```python
from build123d import *

# Parameters (mm, degrees)
F0_R     = 17.018
F0_R_2   = 18.846805
F1_DEPTH = 2
F2_DEPTH = 25
F3_SIZE  = 0.5


with BuildPart() as f1:
    # F0 (on Front) → F1 (new body)
    with BuildSketch(Plane.XZ):
        Circle(F0_R)
        Circle(F0_R_2)
        Circle(F0_R, mode=Mode.SUBTRACT)
    extrude(amount=F1_DEPTH)

    # F0 (on Front) → F2 (cut)
    with BuildSketch(Plane.XZ):
        Circle(F0_R)
    extrude(amount=F2_DEPTH, mode=Mode.SUBTRACT)

    # F3
    f3_edges = [f1.edges().sort_by_distance(p)[0] for p in [
        (-18.846805, 0, 0),
    ]]
    chamfer(f3_edges, length=F3_SIZE)


solid = f1.part
```
Part model, mm, in its own coordinate system. Round coordinates to 2 decimals unless told otherwise and drop trailing zeros. Write each loop counter-clockwise with the first axis right and the second up, starting at its lowest first coordinate (ties: lowest second). Pieces come first, ordered by that corner, then holes. Notation, with made-up numbers: M -12,61 L -7,61 A10 cw -7,79 Z; hole C 35,48.5 d8. An arc over 180 degrees is marked long. One line per question, with ' | ' between items.
(1) Probe line 1 along Z through (x, y) = (0, -0.6); line 2 along X through (y, z) = (-0.75, 7.5); line 3 along Z through (x, y) = (5, -1.4). List the from-to ranges inside material, lowest first.
Answer key:
line 1: z = -18.85 to -17.02, 17.02 to 18.85 | line 2: x = -17.29 to -15.28, 15.28 to 17.29 | line 3: z = -18.17 to -16.27, 16.27 to 18.17
(2) Saw through at C-C on y = -1.3. Write the cut outline in (x, z), then the cut area to 3 significant figures.
Answer key:
outline: C 0,0 d37.69; hole C 0,0 d34.04 | area: 206 mm^2
(3) Two-plate mould, pull along X, no slides. Class faces 1 (the face through (-2.215, -0.986, 16.873)), 2 (the face through (17.976, -1.24, 5.661)), 3 (the face through (-3, -2, 17)): released by +X, released by -X, zero draft, split by the parting line, or undercut.
Answer key:
face 1: undercut | face 2: split by the parting line | face 3: zero draft
(4) Saw through at A-A on z = 0. Write the cut outline in (x, y).
Answer key:
outline: M -18.85,-2 L -17.02,-2 L -17.02,0 L -18.35,0 L -18.85,-0.5 Z; M 17.02,-2 L 18.85,-2 L 18.85,-0.5 L 18.35,0 L 17.02,0 Z
(5) Saw through at B-B on x = 0. Write the cut outline in (y, z), then the cut area to 3 significant figures.
Answer key:
outline: M -2,-18.85 L -0.5,-18.85 L 0,-18.35 L 0,-17.02 L -2,-17.02 Z; M -2,17.02 L 0,17.02 L 0,18.35 L -0.5,18.85 L -2,18.85 Z | area: 7.07 mm^2
(6) Pin check, flat tip, straight feed: pin 1 (1 mm diameter, centred on x = -11.5, y = -1, fed in from +Z). Stop position of the tip, or through.
Answer key:
pin 1: stops at z = 15.3
